For this review, use the dimensioned drawing (mm, ordinates from the lowest corner) and the shaded views. Round coordinates to 2 decimals unless told otherwise and drop trailing zeros. Order: outer loops, then holes, each group sorted by start corner. A loop starts at its lowest first (then second) coordinate and runs counter-clockwise, first axis right, second up. Notation, with made-up numbers: M 42,-36.75 L 50,-36.75 A9 cw 50,-23.75 Z; hole C 55.5,19 d5. An arc over 180 degrees is marked long. Put each result on its own line as item: value.
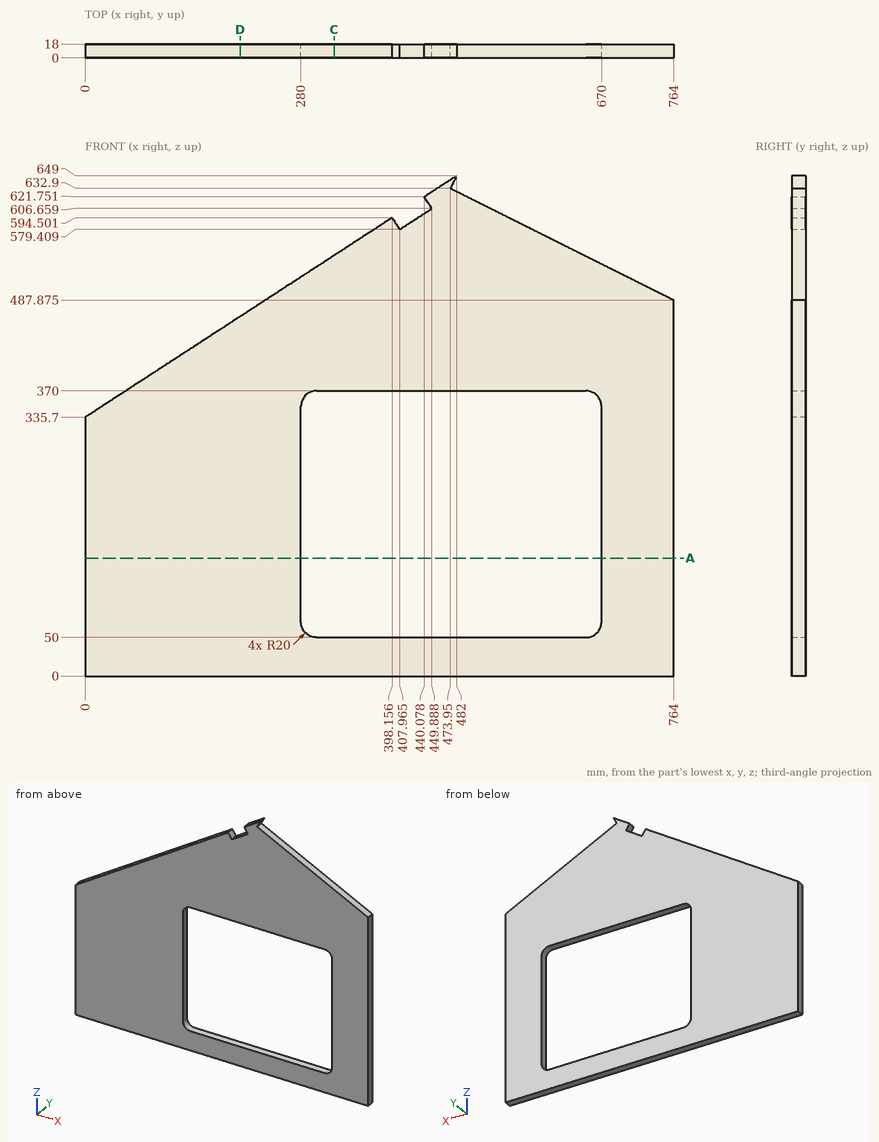
(1) Add section A-A on z = 153. Give the boundary of the cut face in (x, y), then the cut area to 3 significant figures.
A:
outline: M 0,0 L 280,0 L 280,18 L 0,18 Z; M 670,0 L 764,0 L 764,18 L 670,18 Z
area: 6,730 mm2
(2) Insertion check: pin 1 Ø5 at (y, z) = (9.5, 430) entering from -X; pin 2 Ø1.5 at (x, y) = (397, 4) entering from +Z; pin 3 Ø6 at (x, y) = (93.5, 8) entering from +Z (1 decimal). Each pin has a flat end and moves straight along its axis. Give the tip position at first contact, or say it passes through.
A:
pin 1: stops at x = 141.23
pin 2: stops at z = 594.24
pin 3: stops at z = 398.4
(3) To check wall thickness, follow L1, parallel to X at y = 0.5, z = 275.5; L2, parallel to Z at x = 482.5, y = 3.5 (1 decimal); L3, parallel to X at y = 14.5, z = 338 (1 decimal). State the ranges of each line that lie inside material, in increasing order.
A:
L1: x = 0 to 280, 670 to 764
L2: z = 0 to 50, 370 to 628.6
L3: x = 3.5 to 280, 670 to 764
(4) Add section D-D on x = 201. Give the boundary of the cut face in (y, z).
A:
outline: M 0,0 L 18,0 L 18,466.35 L 0,466.35 Z
(5) Add section C-C on x = 323. Give the boundary of the cut face in (y, z), then the cut area to 3 significant figures.
A:
outline: M 0,0 L 18,0 L 18,50 L 0,50 Z; M 0,370 L 18,370 L 18,545.65 L 0,545.65 Z
area: 4,060 mm2
